Source: CAD feature listing. Evaluate the final solid. Frame: model axes, mm. Face numbers are marked on the shaded views. A direction names the side the tool comes from. Give positions to 0.01 mm unless a question says otherwise; leave off trailing zeros. Loops run counter-clockwise (first coordinate to the right, second up) from the corner with the lowest first, then second, coordinate; pieces in that order, holes last. Notation, with made-up numbers: M -27,65.5 L -8,65.5 A25 ccw -8,82.5 Z; hole C 35.5,-35.5 d10. An arc over 180 degrees is marked long. Put each result on its own line as item: value.
from build123d import *

# Parameters (mm, degrees)
SZKIC1_W                         = 48
SZKIC1_H                         = 17.2
DODANIE_WYCI_GNI_CIE1_DEPTH      = 10
SZKIC2_R                         = 1.65
WYTNIJ_WYCI_GNI_CIE1_DEPTH       = 10
SZKIC3_R                         = 2.75
WYTNIJ_WYCI_GNI_CIE2_DEPTH       = 10
SZKIC4_R                         = 1.65
WYTNIJ_WYCI_GNI_CIE3_DEPTH       = 17.2
SZKIC5_W                         = 29
SZKIC5_H                         = 17.2
SZKIC5_R                         = 2.75
DODANIE_WYCI_GNI_CIE2_DEPTH      = 10
SZKIC6_R                         = 1.65
WYTNIJ_WYCI_GNI_CIE4_DEPTH       = 17.2
SZKIC7_W                         = 15
SZKIC7_H                         = 9.959248908
WYTNIJ_WYCI_GNI_CIE5_DEPTH       = 0.1
SFAZOWANIE1_SIZE                 = 5
SZKIC9_R                         = 1.5
WYTNIJ_WYCI_GNI_CIE6_DEPTH       = 10
WYTNIJ_WYCI_GNI_CIE7_DEPTH       = 3.5
DODANIE_WYCI_GNI_CIE3_DEPTH      = 2.5
DODANIE_WYCI_GNI_CIE3_DEPTH_BACK = 1
SZKIC8_W                         = 18
SZKIC8_H                         = 10
WYTNIJ_WYCI_GNI_CIE8_START       = 7.5
SZKIC11_R                        = 1.5
WYTNIJ_WYCI_GNI_CIE8_DEPTH       = 7.5


with BuildPart() as part:
    # Szkic1 → Dodanie-wyciągnięcie1 (new body)
    with BuildSketch(Plane.XY):
        Rectangle(SZKIC1_W, SZKIC1_H)
    extrude(amount=DODANIE_WYCI_GNI_CIE1_DEPTH)

    # Szkic2 → Wytnij-wyciągnięcie1 (cut)
    with BuildSketch(Plane.XY.offset(10)):
        with Locations((-19.5, 0.6)):
            Circle(SZKIC2_R)
        with Locations((19.5, 0.6)):
            Circle(SZKIC2_R)
    extrude(amount=-WYTNIJ_WYCI_GNI_CIE1_DEPTH, mode=Mode.SUBTRACT)

    # Szkic3 → Wytnij-wyciągnięcie2 (cut)
    with BuildSketch(Plane.XY.offset(10)):
        with Locations((0, 0.6)):
            Circle(SZKIC3_R)
    extrude(amount=-WYTNIJ_WYCI_GNI_CIE2_DEPTH, mode=Mode.SUBTRACT)

    # Szkic4 → Wytnij-wyciągnięcie3 (cut)
    with BuildSketch(Plane.XZ.offset(8.6)):
        with Locations(Location((-13, 5, 0), (0, 0, 270))):
            Circle(SZKIC4_R)
        with Locations(Location((13, 5, 0), (0, 0, 270))):
            Circle(SZKIC4_R)
    extrude(amount=-WYTNIJ_WYCI_GNI_CIE3_DEPTH, mode=Mode.SUBTRACT)

    # Szkic5 → Dodanie-wyciągnięcie2 (add)
    with BuildSketch(Plane(origin=(0, 0, 0), x_dir=(-1, 0, 0), z_dir=(0, 0, -1))):
        Rectangle(SZKIC5_W, SZKIC5_H)
        with Locations(Location((0, 0.6, 0), (0, 0, 180))):
            Circle(SZKIC5_R, mode=Mode.SUBTRACT)
    extrude(amount=DODANIE_WYCI_GNI_CIE2_DEPTH)

    # Szkic6 → Wytnij-wyciągnięcie4 (cut)
    with BuildSketch(Plane(origin=(0, 8.6, 0), x_dir=(1, 0, 0), z_dir=(0, 1, 0))):
        with Locations(Location((-10.5, 5, 0), (0, 0, 270))):
            Circle(SZKIC6_R)
        with Locations(Location((10.5, 5, 0), (0, 0, 270))):
            Circle(SZKIC6_R)
    extrude(amount=-WYTNIJ_WYCI_GNI_CIE4_DEPTH, mode=Mode.SUBTRACT)

    # Szkic7 → Wytnij-wyciągnięcie5 (cut)
    with BuildSketch(Plane(origin=(0, 0, -10), x_dir=(-1, 0, 0), z_dir=(0, 0, -1))):
        with Locations((0, -8.6)):
            Rectangle(SZKIC7_W, SZKIC7_H)
    extrude(amount=-WYTNIJ_WYCI_GNI_CIE5_DEPTH, mode=Mode.SUBTRACT)

    # Sfazowanie1
    # the kernel refuses this chamfer: 5 mm, written as the material it takes off along each edge
    with BuildSketch(Plane(origin=(-7.5, -8.6, -9.9), x_dir=(0, -0.027495876610586317, 0.9996219169112968), z_dir=(1, 0, 0))) as sfazowanie1_piece_1_section:
        Polygon((SFAZOWANIE1_SIZE * 0.999621916911, -SFAZOWANIE1_SIZE * 0.0274958766106), (-SFAZOWANIE1_SIZE * 0.0274958766106, -SFAZOWANIE1_SIZE * 0.999621916911), (0, 0), align=None)
    sfazowanie1_piece_1 = extrude(amount=15, mode=Mode.PRIVATE)
    sfazowanie1_piece_1 = split(sfazowanie1_piece_1, bisect_by=Plane(origin=(0, -3.620375546, -8.233305768), z_dir=(0, -1, 0)), keep=Keep.TOP, mode=Mode.PRIVATE)
    add(sfazowanie1_piece_1, mode=Mode.SUBTRACT)

    # Szkic9 → Wytnij-wyciągnięcie6 (cut)
    with BuildSketch(Plane.XZ.offset(8.6)):
        with Locations(Location((0, 5, 0), (0, 0, 270))):
            Circle(SZKIC9_R)
    extrude(amount=-WYTNIJ_WYCI_GNI_CIE6_DEPTH, mode=Mode.SUBTRACT)

    # Szkic10 → Wytnij-wyciągnięcie7 (cut)
    with BuildSketch(Plane.XZ.offset(8.6)):
        Polygon((-2.65, 6.529978213), (-2.65, 10), (2.65, 10), (2.65, 6.529978213), (2.65, 3.470021787), (0, 1.940043573), (-2.65, 3.470021787), align=None)
    extrude(amount=-WYTNIJ_WYCI_GNI_CIE7_DEPTH, mode=Mode.SUBTRACT)

    # Szkic8 → Dodanie-wyciągnięcie3 (add, two sides: drawn at the far end of the back side and taken through both)
    with BuildSketch(Plane.XZ.offset(8.6).offset(-DODANIE_WYCI_GNI_CIE3_DEPTH_BACK)):
        with Locations((0, 5)):
            Rectangle(SZKIC8_W, SZKIC8_H)
    extrude(amount=DODANIE_WYCI_GNI_CIE3_DEPTH + DODANIE_WYCI_GNI_CIE3_DEPTH_BACK)

    # Szkic11 → Wytnij-wyciągnięcie8 (cut)
    with BuildSketch(Plane.XZ.offset(5.1).offset(WYTNIJ_WYCI_GNI_CIE8_START)):
        with Locations(Location((0, 5, 0), (0, 0, 270))):
            Circle(SZKIC11_R)
    extrude(amount=-WYTNIJ_WYCI_GNI_CIE8_DEPTH, mode=Mode.SUBTRACT)


solid = part.part
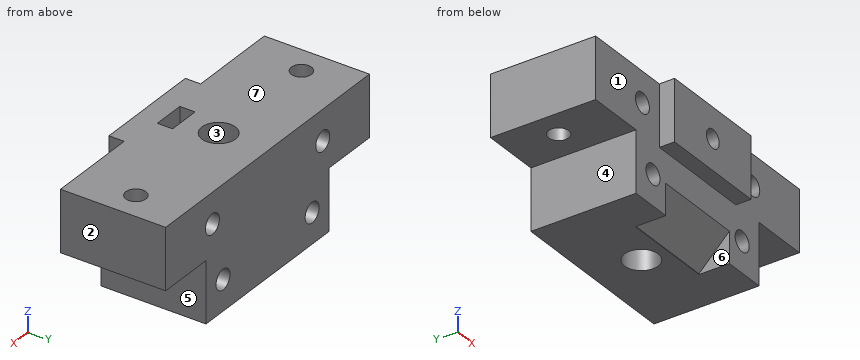
1. Section query D-D (z = 1). Output: boundary loops of the cut face in (x, y).
Found:
outline: M -24,-8.6 L -9,-8.6 L -9,-11.1 L 9,-11.1 L 9,-8.6 L 24,-8.6 L 24,8.6 L -24,8.6 Z; hole C -19.5,0.6 d3.3; hole C 0,0.6 d5.5; hole C 19.5,0.6 d3.3
2. Section query A-A (z = 5). State how many separate pieces and enclosed holes the cut face has, plus the area to 3 significant figures.
Found:
separate pieces: 3
enclosed holes: 2
area: 683 mm^2
3. Contact query for flat-ended pins moving along their axis: P1, Ø2, axis at x = 16.5, y = -8.5, coming from the -Z side; P2, Ø4.5, axis at x = -10.5, z = -5, coming from the +Y side; P3, Ø3, axis at x = 10.5, z = -5, coming from the +Y side; P4, Ø1, axis at x = 13.5, z = -3, coming from the -Y side. Output: stop coordinate, or through.
Found:
P1: z = 0
P2: y = 8.6
P3: through
P4: y = -8.6
4. Access query for the marked faces 4, 5, 6 and 7. Directions: +Z, -Z, +X, -X, +Y, -Y. A direction counts if a zero-diameter tool reaches every point of the face in a straight line with its end or side. Return the directions, or none.
Found:
face 4: -Z, -X, +Y, -Y
face 5: -Z, +X, +Y, -Y
face 6: -Z, -Y
face 7: +Z, +X, -X, +Y, -Y
5. Material intervals for line 1 (X direction, y = -2.75, z = -5); line 2 (X direction, y = -3, z = 5); line 3 (X direction, y = 0.5, z = -2.5), sorted ascending. Write a range as from..to.
Found:
line 1: -14.5..-12.15, -8.85..8.85, 12.15..14.5
line 2: -24..-14.65, -11.35..-1.5, 1.5..11.35, 14.65..24
line 3: -14.5..-2.75, 2.75..14.5
6. Draft query along X for the marked faces 1, 2 and 3. Return one class per face: pulls with the +X half, pulls with the -X half, needs draft (parallel to the pull), parting line crosses it, or undercut.
Found:
face 1: needs draft
face 2: pulls with the +X half
face 3: undercut
7. Section query B-B (x = 19.5). Output: boundary loops of the cut face in (y, z), plus the area to 3 significant figures.
Found:
outline: M -8.6,0 L -1.05,0 L -1.05,10 L -8.6,10 Z; M 2.25,0 L 8.6,0 L 8.6,10 L 2.25,10 Z
area: 139 mm^2
8. Section query C-C (y = 6.5). Output: boundary loops of the cut face in (x, z), plus the area to 3 significant figures.
Found:
outline: M -24,0 L -14.5,0 L -14.5,-10 L 14.5,-10 L 14.5,0 L 24,0 L 24,10 L -24,10 Z; hole C -13,5 d3.3; hole C -10.5,-5 d3.3; hole C 10.5,-5 d3.3; hole C 13,5 d3.3
area: 736 mm^2
